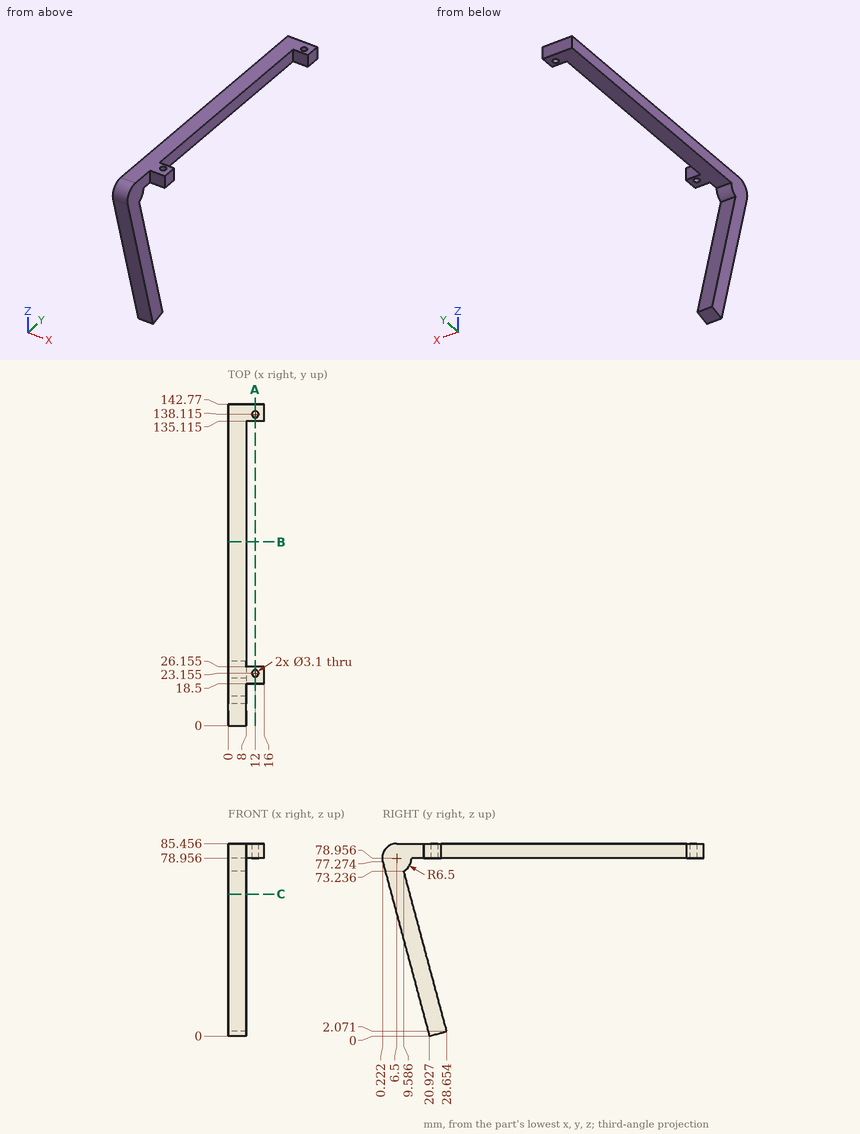
The figure shows three views and two pictorial views of one solid part (mm, origin at its lowest corner). Answer the questions. Give positions to 0.01 mm unless a question says otherwise; leave off trailing zeros. Write each loop counter-clockwise with the first axis right and the second up, starting at its lowest first coordinate (ties: lowest second). Pieces come first, ordered by that corner, then holes. Notation, with made-up numbers: M -15,-5 L 0,-5 A15 ccw 0,0 Z; hole C 69.5,-13 d7. An arc over 180 degrees is marked long. One line per item, written item: value. Start each with the question number.
(1) Find the intervals of material crossed by line 1 (Y direction, x = 12, z = 84.25) (1 decimal); line 2 (Z direction, x = 4, y = 88); line 3 (X direction, y = 24, z = 8), in increasing order.
(2) Find section B-B (y = 81.5). Determine the outline of the cut face in (x, z), plus the area to 3 significant figures.
(3) Find section A-A (x = 12). Determine the outline of the cut face in (y, z) (1 decimal).
(4) Flat-ended cylindrical pins translate along their axes: pin 1 Ø3 at (x, z) = (13, 83.5) entering from -Y; pin 2 Ø1 at (x, y) = (9.5, 48.5) entering from -Z; pin 3 Ø5 at (x, y) = (12, 138.115) entering from -Z; pin 4 Ø1 at (x, z) = (4, 70.5) entering from -Y. Find the tip coordinate at first contact, or state that the pin passes through.
(5) Find section C-C (z = 63). Determine the outline of the cut face in (x, y).
Results below:
1. line 1: y = 18.5 to 21.6, 24.7 to 26.2, 135.1 to 136.6, 139.7 to 142.8
1. line 2: z = 78.96 to 85.46
1. line 3: x = 0 to 8
2. outline: M 0,78.96 L 8,78.96 L 8,85.46 L 0,85.46 Z
2. area: 52.0 mm^2
3. outline: M 18.5,79 L 21.6,79 L 21.6,85.5 L 18.5,85.5 Z; M 24.7,79 L 26.2,79 L 26.2,85.5 L 24.7,85.5 Z; M 135.1,79 L 136.6,79 L 136.6,85.5 L 135.1,85.5 Z; M 139.7,79 L 142.8,79 L 142.8,85.5 L 139.7,85.5 Z
4. pin 1: stops at y = 18.5
4. pin 2: passes through
4. pin 3: stops at z = 78.96
4. pin 4: stops at y = 1.9
5. outline: M 0,4.05 L 8,4.05 L 8,12.33 L 0,12.33 Z
